Source: CAD feature listing. Evaluate the final solid. Frame: model axes, mm. Coordinates: 2 decimals unless noted, no trailing zeros. Order: outer loops, then holes, each group sorted by start corner. A loop starts at its lowest first (then second) coordinate and runs counter-clockwise, first axis right, second up.
```python
from build123d import *

# Parameters (mm, degrees)
ESQUISSE1_W             = 38
ESQUISSE1_H             = 215
BOSS_EXTRU_1_DEPTH      = 6
ESQUISSE2_W             = 15
ESQUISSE2_H             = 23
ENL_V_MAT_EXTRU_1_DEPTH = 219.414743092
ESQUISSE3_W             = 20
ESQUISSE3_H             = 22.5
ENL_V_MAT_EXTRU_2_DEPTH = 7.5
CHANFREIN1_SIZE         = 6
ESQUISSE4_W             = 23
ESQUISSE4_H             = 67
ENL_V_MAT_EXTRU_3_DEPTH = 219.414743092
ESQUISSE5_W             = 7.158748458
ESQUISSE5_H             = 7.5
ENL_V_MAT_EXTRU_4_DEPTH = 219.414743092
ESQUISSE6_R             = 2.5
ENL_V_MAT_EXTRU_5_DEPTH = 10


with BuildPart() as part:
    # Esquisse1 → Boss.-Extru.1 (new body)
    with BuildSketch(Plane.XY):
        with Locations((19, 107.5)):
            Rectangle(ESQUISSE1_W, ESQUISSE1_H)
    extrude(amount=BOSS_EXTRU_1_DEPTH)

    # Esquisse2 → Enlèv. mat.-Extru.1 (cut, through all)
    with BuildSketch(Plane(origin=(0, 0, 0), x_dir=(-1, 0, 0), z_dir=(0, 0, -1))):
        with Locations((-30.5, 87.5)):
            Rectangle(ESQUISSE2_W, ESQUISSE2_H)
    extrude(amount=-ENL_V_MAT_EXTRU_1_DEPTH, mode=Mode.SUBTRACT)

    # Esquisse3 → Enlèv. mat.-Extru.2 (cut)
    with BuildSketch(Plane.XY.offset(6)):
        with Locations((28, 11.25)):
            Rectangle(ESQUISSE3_W, ESQUISSE3_H)
    extrude(amount=-ENL_V_MAT_EXTRU_2_DEPTH, mode=Mode.SUBTRACT)

    # Chanfrein1
    chanfrein1_edges = [part.edges().sort_by_distance(p)[0] for p in [
        (18, 11.25, 6),
    ]]
    chamfer(chanfrein1_edges, length=CHANFREIN1_SIZE - 0.0001)  # a hair under: the kernel refuses the full size

    # Esquisse4 → Enlèv. mat.-Extru.3 (cut, through all)
    with BuildSketch(Plane(origin=(0, 0, 0), x_dir=(-1, 0, 0), z_dir=(0, 0, -1))):
        with Locations((-26.5, 33.5)):
            Rectangle(ESQUISSE4_W, ESQUISSE4_H)
    extrude(amount=-ENL_V_MAT_EXTRU_3_DEPTH, mode=Mode.SUBTRACT)

    # Esquisse5 → Enlèv. mat.-Extru.4 (cut, through all)
    with BuildSketch(Plane(origin=(0, 0, 0), x_dir=(-1, 0, 0), z_dir=(0, 0, -1))):
        with Locations((-11.420625771, 40.825425785)):
            Rectangle(ESQUISSE5_W, ESQUISSE5_H)
    extrude(amount=-ENL_V_MAT_EXTRU_4_DEPTH, mode=Mode.SUBTRACT)

    # Esquisse6 → Enlèv. mat.-Extru.5 (cut)
    with BuildSketch(Plane(origin=(0, 0, 0), x_dir=(-1, 0, 0), z_dir=(0, -1, 0))):
        with Locations(Location((-6, -3, 0), (0, 0, 180))):
            Circle(ESQUISSE6_R)
    extrude(amount=-ENL_V_MAT_EXTRU_5_DEPTH, mode=Mode.SUBTRACT)


solid = part.part
```
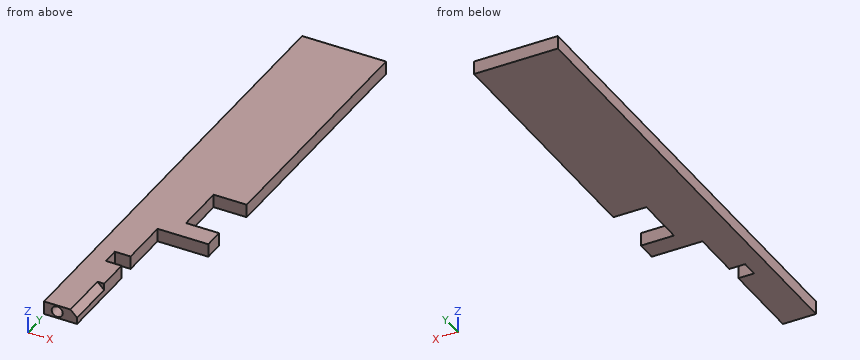
1. Ray query, line 1 (Z direction, x = 6, y = 3.5); line 2 (Y direction, x = 12, z = 3.75); line 3 (Y direction, x = 24.5, z = 0.5). Return the intervals inside material, ascending.
Findings:
line 1: z = 0 to 0.5, 5.5 to 6
line 2: y = 0 to 37.08, 44.58 to 215
line 3: y = 67 to 76, 99 to 215
2. Section query B-B on x = 6. Return loops of the section in (y, z), plus the area to 3 significant figures.
Findings:
outline: (0, 0) - (215, 0) - (215, 6) - (0, 6) - (0, 5.5) - (10, 5.5) - (10, 0.5) - (0, 0.5) - close
area: 1,240 mm2
3. Section query D-D on z = 4.5. Return loops of the section in (x, y), plus the area to 3 significant figures.
Findings:
outline: (0, 0) - (4, 0) - (4, 10) - (8, 10) - (8, 0) - (13.5, 0) - (13.5, 22.5) - (15, 22.5) - (15, 37.08) - (7.84, 37.08) - (7.84, 44.58) - (15, 44.58) - (15, 67) - (38, 67) - (38, 76) - (23, 76) - (23, 99) - (38, 99) - (38, 215) - (0, 215) - close
area: 6,160 mm2
4. Section query A-A on x = 27. Return loops of the section in (y, z).
Findings:
outline: (67, 0) - (76, 0) - (76, 6) - (67, 6) - close; (99, 0) - (215, 0) - (215, 6) - (99, 6) - close
5. Pin query (flat end, axial travel): P1, Ø3, axis at y = 19, z = 3.5, coming from the +X side; P2, Ø1.8, axis at x = 27.5, z = 4.5, coming from the -Y side; P3, Ø1.8, axis at y = 88, z = 4.5, coming from the +X side. Return the tip coordinate at first contact, or that it passes through.
Findings:
P1: stops at x = 15
P2: stops at y = 67
P3: stops at x = 23
6. Section query C-C on y = 86.5. Return loops of the section in (x, z).
Findings:
outline: (0, 0) - (23, 0) - (23, 6) - (0, 6) - close
